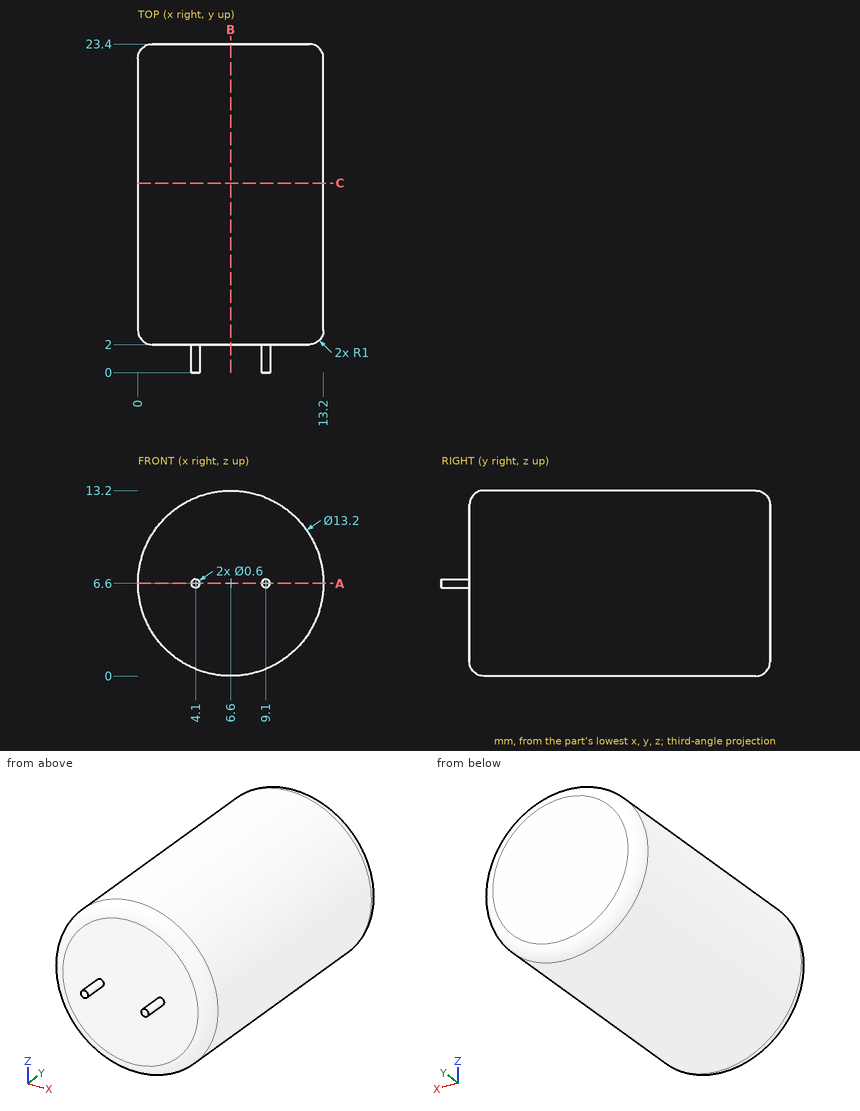
Study the drawing (mm; zero at the part's minimum x, y, z) and answer. Coordinates: 2 decimals unless noted, no trailing zeros. Order: outer loops, then holes, each group sorted by start corner. A loop starts at its lowest first (then second) coordinate and runs counter-clockwise, first axis right, second up. Notation, with made-up numbers: (-16.5, 3.25) -> (41.5, 3.25) arc R16 ccw to (41.5, 21.25) -> close; hole circle Ø4 at (55, 5). An arc over 180 degrees is marked (long way). Answer in a Markdown table with one row per item. Add a question column.
Item 1: Find section A-A (z = 6.6). Write down the section's boundary in (x, y), then the cut area to 3 significant figures.
Item 2: Find section C-C (y = 13.5). Write down the section's boundary in (x, z), then the cut area to 3 significant figures.
Item 3: Each of these flat-tipped pins is pushed along its axis until it touches: P1, Ø1, axis at y = 12, z = 3, coming from the -X side; P2, Ø2, axis at y = 6.5, z = 1.5, coming from the -X side; P3, Ø1.5, axis at x = 8, z = 2.5, coming from the -Y side. Where does it stop, or does it pass through?
Item 4: Find section B-B (x = 6.6). Write down the section's boundary in (y, z), then the cut area to 3 significant figures.
Item 5: Find the intervals of material crossed by L1, parallel to Y at x = 2.75, z = 9.25; L2, parallel to X at y = 3.75, z = 6.75; L3, parallel to X at y = 15.5, z = 9, in increasing order. Write a range as from..to.
Result set:
| question | item | result |
|---|---|---|
| 1 | outline | (0, 3) arc R1 ccw to (1, 2) -> (3.8, 2) -> (3.8, 0) -> (4.4, 0) -> (4.4, 2) -> (8.8, 2) -> (8.8, 0) -> (9.4, 0) -> (9.4, 2) -> (12.2, 2) arc R1 ccw to (13.2, 3) -> (13.2, 22.4) arc R1 ccw to (12.2, 23.4) -> (1, 23.4) arc R1 ccw to (0, 22.4) -> close |
| 1 | area | 284 mm² |
| 2 | outline | circle Ø13.2 at (6.6, 6.6) |
| 2 | area | 137 mm² |
| 3 | P1 | stops at x = 0.77 |
| 3 | P2 | stops at x = 1.43 |
| 3 | P3 | stops at y = 2 |
| 4 | outline | (2, 1) arc R1 ccw to (3, 0) -> (22.4, 0) arc R1 ccw to (23.4, 1) -> (23.4, 12.2) arc R1 ccw to (22.4, 13.2) -> (3, 13.2) arc R1 ccw to (2, 12.2) -> close |
| 4 | area | 282 mm² |
| 5 | L1 | y = 2..23.4 |
| 5 | L2 | x = 0..13.2 |
| 5 | L3 | x = 0.45..12.75 |
